For this review, take the finished solid that the model builds, in its own axes (mm). Face numbers are marked on the shaded views. Give positions to 0.01 mm unless a question says otherwise; leave off trailing zeros. Order: outer loops, then holes, each group sorted by start corner. A loop starts at its lowest first (then second) coordinate and runs counter-clockwise, first axis right, second up. Notation, with made-up numbers: M 33,29.25 L 86,29.25 A21 ccw 86,43.25 Z; hole C 6,61.5 d5. An arc over 180 degrees is marked long. Use CSV: the item, a comma, the result in double quotes. Start each with the question number.
(1) Wall thickness on L1, parallel to X at y = 20, z = 4.05; L2, parallel to Y at x = 19, z = 3.1; L3, parallel to X at y = 0.5, z = 4.15 (3 decimals): over which ranges is each line inside the solid? List them lowest first. Write a range as from..to.
(2) Consider section A-A (y = 0). Write out the cut boundary in (x, z).
(3) Clearance check with flat-ended pins moving along their axes: P1, Ø2, axis at x = 17.5, z = 1, coming from the -Y side; P2, Ø1.5, axis at x = 1, z = 2, coming from the +Y side. State where each tip first meets the part, or that it passes through.
(4) Draft analysis for pull direction X (two halves, no side actions). For the marked faces 1, 2 and 3, state which applies: pulls with the +X half, pulls with the -X half, needs draft (parallel to the pull), parting line crosses it, or undercut.
(5) Consider section C-C (y = 9.5). Write out the cut boundary in (x, z).
(6) Consider section D-D (z = 0.8). Give the number of separate pieces and of enclosed holes in the cut face, and give its area (3 significant figures).
Autodesk Fusion 360 part; units mm, degrees
sketch "スケッチ1" plane through (0, 0, 0) normal (0, 0, 1) x (1, 0, 0)
  circle A0 centre (0, 0) radius 25
  circle A1 centre (0, 0) radius 27.5
  dimension "d1" = 55
extrude "押し出し1" add sketch "スケッチ1" along normal blind 5
sketch "スケッチ2" plane through (0, 0, 5) normal (0, 0, 1) x (-1, 0, 0)
  circle A0 centre (0, 0) radius 25
  circle A1 centre (0, 0) radius 27.5
  circle A2 centre (0, 0) radius 30
extrude "押し出し2" add sketch "スケッチ2" against normal blind 5 contours A2
sketch "スケッチ3" plane through (0, 0, 5) normal (0, 0, 1) x (-1, 0, 0)
  circle A0 centre (0, 0) radius 30
  circle A1 centre (0, 0) radius 25
  circle A2 centre (0, 0) radius 27.5
  circle A3 centre (-27.5, 0) radius 1.5
  circle A4 centre (-19.4454, -19.4454) radius 1.5
  circle A5 centre (0, -27.5) radius 1.5
  circle A6 centre (19.4454, -19.4454) radius 1.5
  circle A7 centre (27.5, 0) radius 1.5
  circle A8 centre (19.4454, 19.4454) radius 1.5
  circle A9 centre (0, 27.5) radius 1.5
  circle A10 centre (-19.4454, 19.4454) radius 1.5
  dimension "d6" = 55
  dimension "d7" = 3
  dimension "d9" = 360
extrude "押し出し3" cut sketch "スケッチ3" against normal blind 6 contours A2 A7 | A2 A7 | A2 A8 | A2 A8 | A2 A6 | A2 A6 | A2 A9 | A2 A9 | A2 A5 | A2 A5 | A2 A10 | A2 A10 | A2 A4 | A2 A4 | A2 A3 | A2 A3
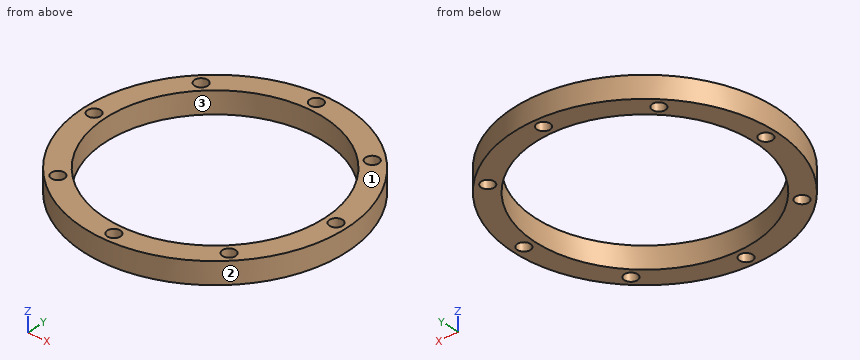
Check result:
1,L1,"x = -22.36..-20.84, -18.05..-15, 15..18.05, 20.84..22.36"
1,L2,"y = -23.22..-20.88, -18.01..-16.25, 16.25..18.01, 20.88..23.22"
1,L3,"x = -29.996..-28.914, -26.086..-24.995, 24.995..26.086, 28.914..29.996"
2,outline,"M -30,0 L -29,0 L -29,5 L -30,5 Z; M -26,0 L -25,0 L -25,5 L -26,5 Z; M 25,0 L 26,0 L 26,5 L 25,5 Z; M 29,0 L 30,0 L 30,5 L 29,5 Z"
3,P1,"stops at y = -25.05"
3,P2,"stops at y = 30"
4,face 1,"needs draft"
4,face 2,"parting line crosses it"
4,face 3,"undercut"
5,outline,"M -28.46,0 L -23.12,0 L -23.12,5 L -28.46,5 Z; M 23.12,0 L 28.46,0 L 28.46,5 L 23.12,5 Z"
6,separate pieces,"1"
6,enclosed holes,"9"
6,area,"807 mm^2"
